from build123d import *

# Parameters (mm, degrees)
F2_R     = 6.35
F3_DEPTH = 19.051


with BuildPart() as f1:
    # F0 (on Right) → F1 (revolve)
    with BuildSketch(Plane.YZ):
        with BuildLine():
            Line((0, 19.05), (53.848, 19.05))
            Line((53.848, 19.05), (53.848, 76.2))
            Line((53.848, 76.2), (37.846, 76.2))
            ThreePointArc((37.846, 76.2), (35.690739, 75.307261), (34.798, 73.152))
            Line((34.798, 73.152), (34.798, 44.196))
            ThreePointArc((34.798, 44.196), (33.905261, 42.040739), (31.75, 41.148))
            Line((31.75, 41.148), (3.048, 41.148))
            ThreePointArc((3.048, 41.148), (0.892739, 40.255261), (0, 38.1))
            Line((0, 38.1), (0, 19.05))
        make_face()
    revolve(axis=Axis((0, 35.464443, 0), (0, 1, 0)))

    # F2 (on face) → F3 (cut, through all)
    with BuildSketch(Plane.XZ.offset(-34.798)):
        with Locations((0, 53.848)):
            Circle(F2_R)
        with Locations((53.848, 0)):
            Circle(F2_R)
        with Locations((0, -53.848)):
            Circle(F2_R)
        with Locations((-53.848, 0)):
            Circle(F2_R)
    extrude(amount=-F3_DEPTH, mode=Mode.SUBTRACT)


solid = f1.part
Input: part model. Units: mm. Frame: model coordinates. Coordinates: 2 decimals unless noted, no trailing zeros. Order: outer loops, then holes, each group sorted by start corner. A loop starts at its lowest first (then second) coordinate and runs counter-clockwise, first axis right, second up. Notation, with made-up numbers: M 68,44.25 L 118,44.25 A30 ccw 118,72.25 Z; hole C 37,12.5 d5. An arc over 180 degrees is marked long. Write item = value, one per line. Start each with the question number.
(1) Section A-A on x = 0. Output: boundary loops of the cut face in (y, z), and give its area (3 significant figures).
(2) Section C-C on y = 19. Output: boundary loops of the cut face in (x, z).
(3) First-contact query: P1, Ø1, axis at y = 18.5, z = -26.5, coming from the -X side; P2, Ø1.5, axis at x = 1, y = 24, coming from the -Z side; P3, Ø20.5, axis at x = -53.848, z = 0, coming from the -Y side. Flat tips, straight axial feed; report the tip coordinate or a pass-through.
(4) Line query: line 1 along X through (y, z) = (29, 0); line 2 along X through (y, z) = (49.5, 4.5); line 3 along Y through (x, z) = (48, -37.5). Output: solid intervals per line, ascending. Write a range as [from, to].
(5) Pull-direction query (X, two-part tool) for faces 1 (the cylindrical face through (40.798, 17.198, -5.357)), 2 (the cylindrical face through (-0.827, 44.19, 60.144)), 3 (the flat face through (-31.5, 34.798, 31.5)), 4 (the cylindrical face through (-11.59, 27.3, -15.12)); classes: released by +X, released by -X, zero draft, split by the parting line, or undercut.
(6) Section B-B on z = 0. Output: boundary loops of the cut face in (x, y), and give its area (3 significant figures).
(7) Section D-D on y = 48. Output: boundary loops of the cut face in (x, z).
Result set:
q1.outline = M 0,-38.1 A3.05 ccw 3.05,-41.15 L 31.75,-41.15 A3.05 cw 34.8,-44.2 L 34.8,-47.5 L 53.85,-47.5 L 53.85,-19.05 L 0,-19.05 Z; M 0,19.05 L 53.85,19.05 L 53.85,47.5 L 34.8,47.5 L 34.8,44.2 A3.05 cw 31.75,41.15 L 3.05,41.15 A3.05 ccw 0,38.1 Z; M 34.8,-73.15 A3.05 ccw 37.85,-76.2 L 53.85,-76.2 L 53.85,-60.2 L 34.8,-60.2 Z; M 34.8,60.2 L 53.85,60.2 L 53.85,76.2 L 37.85,76.2 A3.05 ccw 34.8,73.15 Z
q1.area = 3,230 mm²
q2.outline = C 0,0 d82.3; hole C 0,0 d38.1
q3.P1 = -31.89
q3.P2 = -41.15
q3.P3 = 34.74
q4.line_1 = [-41.15, -19.05], [19.05, 41.15]
q4.line_2 = [-76.07, -58.33], [-49.37, -18.51], [18.51, 49.37], [58.33, 76.07]
q4.line_3 = [34.8, 53.85]
q5.face_1 = split by the parting line
q5.face_2 = undercut
q5.face_3 = zero draft
q5.face_4 = undercut
q6.outline = M -76.2,37.85 A3.05 ccw -73.15,34.8 L -60.2,34.8 L -60.2,53.85 L -76.2,53.85 Z; M -47.5,34.8 L -44.2,34.8 A3.05 cw -41.15,31.75 L -41.15,3.05 A3.05 ccw -38.1,0 L -19.05,0 L -19.05,53.85 L -47.5,53.85 Z; M 19.05,0 L 38.1,0 A3.05 ccw 41.15,3.05 L 41.15,31.75 A3.05 cw 44.2,34.8 L 47.5,34.8 L 47.5,53.85 L 19.05,53.85 Z; M 60.2,34.8 L 73.15,34.8 A3.05 ccw 76.2,37.85 L 76.2,53.85 L 60.2,53.85 Z
q6.area = 3,230 mm²
q7.outline = C 0,0 d152.4; hole C -53.85,0 d12.7; hole C 0,0 d38.1; hole C 0,-53.85 d12.7; hole C 0,53.85 d12.7; hole C 53.85,0 d12.7
